Read the model definition and answer for the solid it produces. Units are mm, in the model's axes. A direction names the side the tool comes from. Coordinates: 2 decimals unless noted, no trailing zeros. Write each loop counter-clockwise with the first axis right and the second up, starting at its lowest first coordinate (ties: lowest second). Pieces come first, ordered by that corner, then holes. Notation, with made-up numbers: (-17.75, 32.25) - (8.25, 32.25) arc R9 cw to (8.25, 44.25) - close; hole circle Ø4 at (79, 53.5). An arc over 180 degrees is marked (long way). Use a Markdown table: item, result.
from build123d import *

# Parameters (mm, degrees)
F0_R     = 40
F1_DEPTH = 10
F2_R     = 7
F3_R     = 10.625
F4_DEPTH = 10


with BuildPart() as f1:
    # F0 (on Top) → F1 (new body)
    with BuildSketch(Plane.XY):
        Circle(F0_R)
    extrude(amount=F1_DEPTH)

    # F2
    f2_edges = [f1.edges().sort_by_distance(p)[0] for p in [
        (-40, 0, 10),
    ]]
    fillet(f2_edges, radius=F2_R)

    # F3 (on face) → F4 (join)
    with BuildSketch(Plane.XY.offset(10)):
        Circle(F3_R)
    extrude(amount=F4_DEPTH)


solid = f1.part
(1) For faces 1 (the cylindrical face through (-8.43, -6.47, 14.93)), 2 (the flat face through (0, 0, 20)), determine the directions among +Z, -Z, +X, -X, +Y, -Y from which every point of the face is accessible in a straight line to the end or side of a thin tool.
Report:
| item | result |
|---|---|
| face 1 | +Z |
| face 2 | +Z, +X, -X, +Y, -Y |
(2) Each of these flat-tipped pins is pushed along its axis until it touches: P1, Ø10, axis at x = 12, z = 17.5, coming from the -Y side; P2, Ø2, axis at x = 5, z = 7.5, coming from the -Y side; P3, Ø2, axis at y = 9.5, z = 2.5, coming from the -X side; P4, Ø2, axis at y = 21, z = 12.5, coming from the +X side. Where does it stop, or does it pass through?
Report:
| item | result |
|---|---|
| P1 | stops at y = -7.99 |
| P2 | stops at y = -38.75 |
| P3 | stops at x = -39.09 |
| P4 | passes through |
(3) A cutting plane is placed at A-A, the plane x = 0. Write down the section's boundary in (y, z) (3 decimals).
Report:
| item | result |
|---|---|
| outline | (-40, 0) - (40, 0) - (40, 3) arc R7 ccw to (33, 10) - (10.625, 10) - (10.625, 20) - (-10.625, 20) - (-10.625, 10) - (-33, 10) arc R7 ccw to (-40, 3) - close |
(4) A cutting plane is placed at D-D, the plane z = 8.5. Write down the section's boundary in (x, y), and give its area (3 significant figures).
Report:
| item | result |
|---|---|
| outline | circle Ø74.66 at (0, 0) |
| area | 4,380 mm² |
(5) Straight lines are drawn through the part: L1, parallel to Z at x = -8, y = 27.5; L2, parallel to Y at x = -22.5, z = 3.75; L3, parallel to X at y = 33, z = 3.5. For each, find the intervals that lie inside material, in ascending order.
Report:
| item | result |
|---|---|
| L1 | z = 0 to 10 |
| L2 | y = -33.02 to 33.02 |
| L3 | x = -22.57 to 22.57 |
(6) A cutting plane is placed at C-C, the plane z = 18.75. Write down the section's boundary in (x, y) (3 decimals), and give its area (3 significant figures).
Report:
| item | result |
|---|---|
| outline | circle Ø21.25 at (0, 0) |
| area | 355 mm² |
